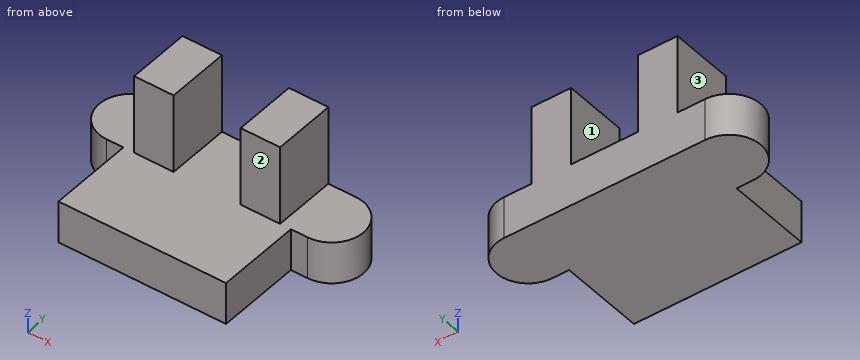
from build123d import *

# Parameters (mm, degrees)
BOSS_EXTRUDE1_DEPTH = 4.27
SKETCH3_W           = 4
SKETCH3_H           = 6.4
BOSS_EXTRUDE2_DEPTH = 8


with BuildPart() as part:
    # Sketch2 → Boss-Extrude1 (new body)
    with BuildSketch(Plane.XY):
        with BuildLine():
            Line((0, 3.2), (20.4, 3.2))
            ThreePointArc((20.4, 3.2), (23.6, 0), (20.4, -3.2))
            Line((20.4, -3.2), (18.7, -3.2))
            Line((18.7, -3.2), (18.7, -11.8))
            Line((18.7, -11.8), (1.7, -11.8))
            Line((1.7, -11.8), (1.7, -3.2))
            Line((1.7, -3.2), (0, -3.2))
            ThreePointArc((0, -3.2), (-3.2, 0), (0, 3.2))
        make_face()
    extrude(amount=BOSS_EXTRUDE1_DEPTH)

    # Sketch3 → Boss-Extrude2 (add)
    with BuildSketch(Plane.XY.offset(4.27)):
        with Locations((4.8, 0)):
            Rectangle(SKETCH3_W, SKETCH3_H)
        with Locations((15.6, 0)):
            Rectangle(SKETCH3_W, SKETCH3_H)
    extrude(amount=BOSS_EXTRUDE2_DEPTH)


solid = part.part
CAD build for the part. Positions are in the model's coordinates, mm. Face numbers are marked on the shaded views. A direction names the side the tool comes from. Give positions to 0.01 mm unless a question says otherwise; leave off trailing zeros. Order: outer loops, then holes, each group sorted by start corner. A loop starts at its lowest first (then second) coordinate and runs counter-clockwise, first axis right, second up. Notation, with made-up numbers: (-30.75, 73.25) -> (-0.75, 73.25) arc R27 cw to (-0.75, 103.25) -> close; hole circle Ø9 at (80.25, 4). An arc over 180 degrees is marked (long way). Return JSON: item names as keys, results as strings.
Q1. Saw through at D-D (z = 3.75). Write the cut outline in (x, y).
Working result:
{"outline": "(0, -3.2) -> (1.7, -3.2) -> (1.7, -11.8) -> (18.7, -11.8) -> (18.7, -3.2) -> (20.4, -3.2) arc R3.2 ccw to (20.4, 3.2) -> (0, 3.2) arc R3.2 ccw to start"}
Q2. Saw through at A-A (z = 7.5). Write the cut outline in (x, y).
Working result:
{"outline": "(2.8, -3.2) -> (6.8, -3.2) -> (6.8, 3.2) -> (2.8, 3.2) -> close; (13.6, -3.2) -> (17.6, -3.2) -> (17.6, 3.2) -> (13.6, 3.2) -> close"}
Q3. Saw through at B-B (y = 0). Write the cut outline in (x, z), then the cut area to 3 significant figures.
Working result:
{"outline": "(-3.2, 0) -> (23.6, 0) -> (23.6, 4.27) -> (17.6, 4.27) -> (17.6, 12.27) -> (13.6, 12.27) -> (13.6, 4.27) -> (6.8, 4.27) -> (6.8, 12.27) -> (2.8, 12.27) -> (2.8, 4.27) -> (-3.2, 4.27) -> close", "area": "178 mm²"}
Q4. Saw through at C-C (x = 14.75). Write the cut outline in (y, z).
Working result:
{"outline": "(-11.8, 0) -> (3.2, 0) -> (3.2, 12.27) -> (-3.2, 12.27) -> (-3.2, 4.27) -> (-11.8, 4.27) -> close"}
Q5. Flat gauge pins, fed straight in: pin 1 (7 mm diameter, centred on y = -1, z = 10, fed in from -X); pin 2 (4 mm diameter, centred on x = 17, y = -5, fed in from +Z); pin 3 (7 mm diameter, centred on y = -1.5, z = 9, fed in from +X); pin 4 (0.8 mm diameter, centred on x = 1, z = 2, fed in from -Y). Where does each tip first touch, or does it go through?
Working result:
{"pin 1": "x = 2.8", "pin 2": "z = 12.27", "pin 3": "x = 17.6", "pin 4": "y = -3.2"}
Q6. Drill centre lines: line 1 (X direction, y = -1.5, z = 10); line 2 (Y direction, x = 15.75, z = 6); line 3 (Z direction, x = 11.25, y = -10.5). Where is each one in solid material? Low to high.
Working result:
{"line 1": "2.8 to 6.8, 13.6 to 17.6", "line 2": "-3.2 to 3.2", "line 3": "0 to 4.27"}
Q7. Which spindle directions (+Z, -Z, +X, -X, +Y, -Y) get a long thin tool onto all of the face, cutting with end or side? Do the marked faces 1, 2 and 3. Say none if no direction does.
Working result:
{"face 1": "+Z, +Y, -Y", "face 2": "+Z, +X, -X, -Y", "face 3": "+Z, -X, +Y, -Y"}
